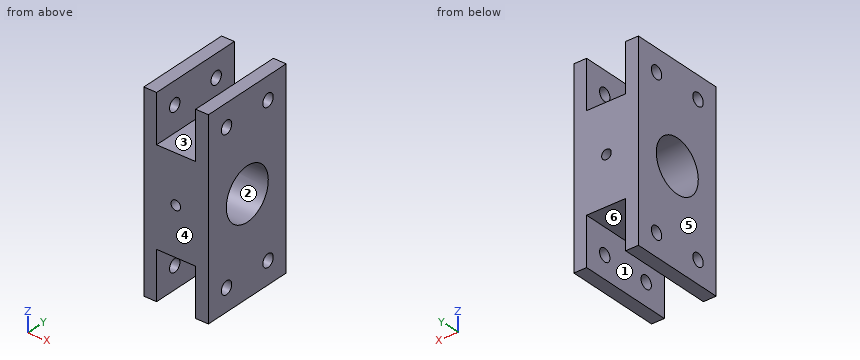
from build123d import *

# Parameters (mm, degrees)
SKETCH_1_W          = 60
SKETCH_1_H          = 30
SKETCH_1_R          = 2
EXTRUDE_1_DEPTH     = 20.2
SKETCH_2_W          = 12.2
SKETCH_2_H          = 15
CUT_EXTRUDE_1_DEPTH = 47.989786124
SKETCH_3_R          = 8.1
CUT_EXTRUDE_2_DEPTH = 40.154054707
SKETCH_4_R          = 1.5
CUT_EXTRUDE_3_DEPTH = 47.989786124


with BuildPart() as part:
    # 스케치1 → 보스-돌출1 (new body)
    with BuildSketch(Plane(origin=(0, 0, 0), x_dir=(0, 0, -1), z_dir=(1, 0, 0))):
        Rectangle(SKETCH_1_W, SKETCH_1_H)
        with Locations((-23, 8)):
            Circle(SKETCH_1_R, mode=Mode.SUBTRACT)
        with Locations(Location((-23, -8, 0), (0, 0, 180))):
            Circle(SKETCH_1_R, mode=Mode.SUBTRACT)
        with Locations((23, -8)):
            Circle(SKETCH_1_R, mode=Mode.SUBTRACT)
        with Locations(Location((23, 8, 0), (0, 0, 180))):
            Circle(SKETCH_1_R, mode=Mode.SUBTRACT)
    extrude(amount=EXTRUDE_1_DEPTH)

    # 스케치2 → 컷-돌출1 (cut, through all)
    with BuildSketch(Plane(origin=(0, 15, 0), x_dir=(1, 0, 0), z_dir=(0, 1, 0))):
        with Locations((10.1, 22.5)):
            Rectangle(SKETCH_2_W, SKETCH_2_H)
        with Locations((10.1, -22.5)):
            Rectangle(SKETCH_2_W, SKETCH_2_H)
    extrude(amount=-CUT_EXTRUDE_1_DEPTH, mode=Mode.SUBTRACT)

    # 스케치3 → 컷-돌출2 (cut, through all)
    with BuildSketch(Plane.ZY):
        Circle(SKETCH_3_R)
    extrude(amount=-CUT_EXTRUDE_2_DEPTH, mode=Mode.SUBTRACT)

    # 스케치4 → 컷-돌출3 (cut, through all)
    with BuildSketch(Plane(origin=(0, 15, 0), x_dir=(1, 0, 0), z_dir=(0, 1, 0))):
        with Locations(Location((10, 0, 0), (0, 0, 270))):
            Circle(SKETCH_4_R)
    extrude(amount=-CUT_EXTRUDE_3_DEPTH, mode=Mode.SUBTRACT)


solid = part.part
Verification items for the finished model (mm, model axes). Face numbers are marked on the shaded views. A direction names the side the tool comes from. Give positions to 0.01 mm unless a question says otherwise; leave off trailing zeros. Loops run counter-clockwise (first coordinate to the right, second up) from the corner with the lowest first, then second, coordinate; pieces in that order, holes last.
1. Go/stop test with flat-tipped pins: P1, Ø3.5, axis at y = 8, z = -23, coming from the -X side; P2, Ø6, axis at x = 12.5, y = 0, coming from the +Z side. Record where each tip stops, or that it passes through.
Derived:
P1: passes through
P2: stops at z = 15
2. Cross-section at A-A on x = 10. Record the cut outline in (y, z), and give its area (3 significant figures).
Derived:
outline: (-15, -15) - (15, -15) - (15, -1.5) - (7.96, -1.5) arc R8.1 cw to (-7.96, -1.5) - (-15, -1.5) - close; (-15, 1.5) - (-7.96, 1.5) arc R8.1 cw to (7.96, 1.5) - (15, 1.5) - (15, 15) - (-15, 15) - close
area: 652 mm2
3. Cross-section at D-D on x = 1.5. Record the cut outline in (y, z).
Derived:
outline: (-15, -30) - (15, -30) - (15, 30) - (-15, 30) - close; hole circle Ø4 at (-8, -23); hole circle Ø4 at (-8, 23); hole circle Ø16.2 at (0, 0); hole circle Ø4 at (8, -23); hole circle Ø4 at (8, 23)
4. Material ranges on probe 1 along Y at (x, z) = (18.4, 23); probe 2 along Z at (x, y) = (10, 11.5); probe 3 along X at (y, z) = (12, 0), recorded low to high.
Derived:
probe 1: y = -15 to -10, -6 to 6, 10 to 15
probe 2: z = -15 to -1.5, 1.5 to 15
probe 3: x = 0 to 8.5, 11.5 to 20.2
5. Cross-section at C-C on y = 9. Count the separate pieces of the cut face and the enclosed holes in it, and give its area (3 significant figures).
Derived:
separate pieces: 5
enclosed holes: 1
area: 784 mm2
6. Tool access check on the marked faces 1, 2 and 3. Record the directions out of +Z, -Z, +X, -X, +Y, -Y that give a thin tool (end or side, any length) a straight path to the whole face; none if there is none.
Derived:
face 1: -Z, +Y, -Y
face 2: +X, -X
face 3: +Z, +Y, -Y
7. Release check for a two-part mould opening along X. For the marked faces 4, 5 and 6 record: +X half, -X half, draft (parallel to the pull), parting line (faces both ways), or undercut.
Derived:
face 4: draft
face 5: -X half
face 6: undercut
8. Cross-section at B-B on z = 0. Record the cut outline in (x, y), and give its area (3 significant figures).
Derived:
outline: (0, -15) - (8.5, -15) - (8.5, -8.1) - (0, -8.1) - close; (0, 8.1) - (8.5, 8.1) - (8.5, 15) - (0, 15) - close; (11.5, -15) - (20.2, -15) - (20.2, -8.1) - (11.5, -8.1) - close; (11.5, 8.1) - (20.2, 8.1) - (20.2, 15) - (11.5, 15) - close
area: 237 mm2
